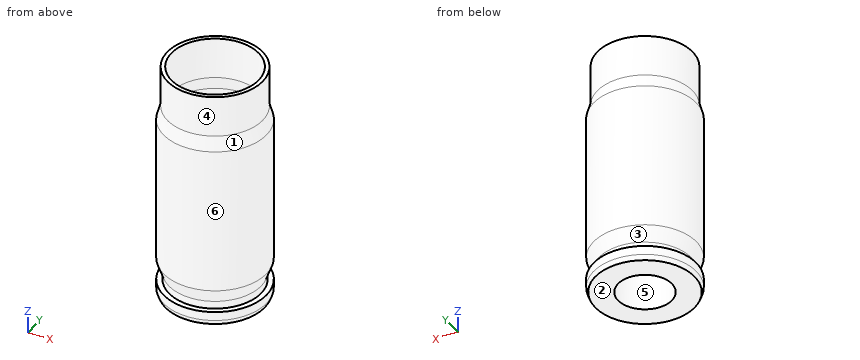
from build123d import *


with BuildPart() as f1:
    # F0 (on Front) → F1 (revolve)
    with BuildSketch(Plane.XZ):
        Polygon((2.2225, 3.048), (2.2225, 0), (4.106582, 0), (4.2545, 0.4064), (4.2545, 1.143), (3.81, 1.143), (3.81, 1.778), (4.2545, 2.999254), (4.2545, 15.1384), (3.937, 16.3068), (3.937, 19.7104), (3.6068, 19.7104), (3.6068, 16.3068), (3.9243, 15.1384), (3.8735, 3.81), (0.9398, 3.81), (0.9398, 3.048), align=None)
    revolve(axis=Axis((0, 0, 11.499301), (0, 0, 1)))


with BuildPart() as f2_1:
    # F2: copy of F1
    add(f1.part)


solid = f1.part
Geometry check sheet. Reference: the model listing, model coordinates, mm. Face numbers are marked on the shaded views. A direction names the side the tool comes from. Give positions to 0.01 mm unless a question says otherwise; leave off trailing zeros. Loops run counter-clockwise (first coordinate to the right, second up) from the corner with the lowest first, then second, coordinate; pieces in that order, holes last.
(1) Section check B-B on z = 16. Record the cut outline in (x, y), then the cut area to 3 significant figures.
From the geometry:
outline: circle Ø8.04 at (0, 0); hole circle Ø7.38 at (0, 0)
area: 8.00 mm2
(2) Release check for a two-part mould opening along Z. For the marked faces 1, 2 and 3 record: released by +Z, released by -Z, zero draft, split by the parting line, or undercut.
From the geometry:
face 1: released by +Z
face 2: released by -Z
face 3: undercut
(3) Depth check by flat-ended pin: pin 1 Ø4 at (x, y) = (3, 0) entering from -Z; pin 2 Ø2 at (x, y) = (-1, 0.5) entering from -Z; pin 3 Ø2 at (y, z) = (-2.5, 13.5) entering from -X; pin 4 Ø4 at (x, z) = (2.5, 8.5) entering from +Y (3 decimals). Enter the tip coordinate at first touch or a pass-through.
From the geometry:
pin 1: stops at z = 0
pin 2: stops at z = 3.05
pin 3: stops at x = -3.98
pin 4: stops at y = 4.225
(4) Thickness scan on L1, parallel to Y at x = 0, z = 3.35; L2, parallel to Z at x = 0.5, y = 2.5; L3, parallel to Y at x = -0.5, z = 6.25. Record the ranges inside material, lowest first.
From the geometry:
L1: y = -4.25 to -0.94, 0.94 to 4.25
L2: z = 0 to 3.81
L3: y = -4.23 to -3.85, 3.85 to 4.23
(5) Set-up check for the marked faces 4, 5 and 6: record each of +Z, -Z, +X, -X, +Y, -Y from which the full face is reachable in a straight line by a thin tool's end or side.
From the geometry:
face 4: +Z
face 5: -Z
face 6: +Z, -Z
(6) Section check A-A on z = 18.5. Record the cut outline in (x, y), then the cut area to 3 significant figures.
From the geometry:
outline: circle Ø7.87 at (0, 0); hole circle Ø7.21 at (0, 0)
area: 7.83 mm2
